Part model, mm, in its own coordinate system. Give positions to 0.01 mm unless a question says otherwise; leave off trailing zeros. Order: outer loops, then holes, each group sorted by start corner. A loop starts at its lowest first (then second) coordinate and runs counter-clockwise, first axis right, second up. Notation, with made-up numbers: M -21.5,0.25 L 1.5,0.25 A27 cw 1.5,26.25 Z; hole C 59.5,51 d5. An arc over 180 degrees is marked long. Answer as a JSON object with one key per item and string values.
from build123d import *

# Parameters (mm, degrees)
F0_R           = 6
F1_DEPTH       = 60
F3_D           = 6.3
F3_CSINK_D     = 13.44
F3_CSINK_ANGLE = 90


with BuildPart() as f1:
    # F0 (on Front) → F1 (new body, symmetric)
    with BuildSketch(Plane.XZ):
        with Locations((-6, 0)):
            Circle(F0_R)
    extrude(amount=F1_DEPTH, both=True)

    # F3 (through all)
    with Locations(Plane.YZ):
        with Locations((12.5, 0), (-12.5, 0)):
            CounterSinkHole(F3_D / 2, F3_CSINK_D / 2, counter_sink_angle=F3_CSINK_ANGLE)


solid = f1.part
1. Pin check, flat tips, straight feed: P1, Ø5, axis at x = -2.5, y = 31.5, coming from the +Z side; P2, Ø7, axis at y = -12.5, z = 0, coming from the +X side; P3, Ø1.5, axis at x = -3.5, y = 45.5, coming from the -Z side. Stop position of each tip, or through.
Worked answers:
{"P1": "stops at z = 5.92", "P2": "stops at x = -3.22", "P3": "stops at z = -5.74"}
2. Two-plate mould, pull along Z, no slides. Class faces 1 (the cylindrical face through (-7.848, -9.353, 0.138)), 2 (the flat face through (-6, 60, 0)), 3 (the cylindrical face through (-12, -1, 0)): +Z half, -Z half, draft (parallel to the pull), parting line (faces both ways), or undercut.
Worked answers:
{"face 1": "undercut", "face 2": "draft", "face 3": "parting line"}
3. Probe line 1 along Y through (x, z) = (-9.75, 0); line 2 along Z through (x, y) = (-6.5, 12.5); line 3 along Y through (x, z) = (-9, 2). List the from-to ranges inside material, lowest first.
Worked answers:
{"line 1": "y = -60 to -15.65, -9.35 to 9.35, 15.65 to 60", "line 2": "z = -5.98 to -3.15, 3.15 to 5.98", "line 3": "y = -60 to -14.93, -10.07 to 10.07, 14.93 to 60"}
4. Cut at B-B on x = -6. Give the cut face in (y, z), plus the area to 3 significant figures.
Worked answers:
{"outline": "M -60,-6 L 60,-6 L 60,6 L -60,6 Z; hole C -12.5,0 d6.3; hole C 12.5,0 d6.3", "area": "1,380 mm^2"}
5. Cut at C-C on y = 12.5. Give the cut face in (x, z), plus the area to 3 significant figures.
Worked answers:
{"outline": "M -11.11,-3.15 A6 ccw -2.13,-4.59 L -3.57,-3.15 Z; M -11.11,3.15 L -3.57,3.15 L -2.13,4.59 A6 ccw Z", "area": "37.1 mm^2"}
6. Cut at D-D on y = 35.5. Give the cut face in (x, z).
Worked answers:
{"outline": "C -6,0 d12"}
7. Cut at A-A on z = 0. Give the cut face in (x, y), plus the area to 3 significant figures.
Worked answers:
{"outline": "M -12,-60 L 0,-60 L 0,-19.22 L -3.57,-15.65 L -12,-15.65 Z; M -12,-9.35 L -3.57,-9.35 L 0,-5.78 L 0,5.78 L -3.57,9.35 L -12,9.35 Z; M -12,15.65 L -3.57,15.65 L 0,19.22 L 0,60 L -12,60 Z", "area": "1,260 mm^2"}
